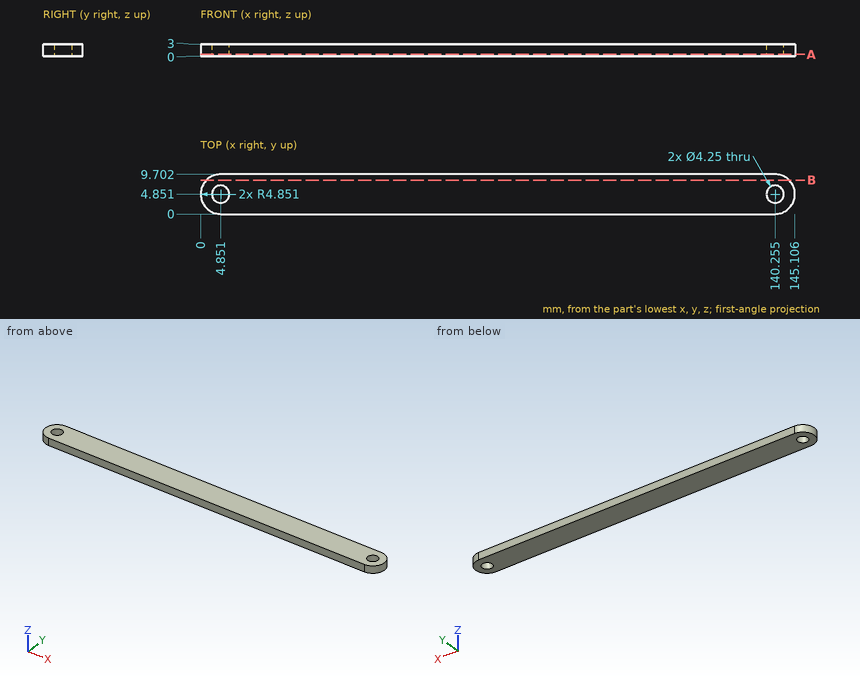
Print and shaded views of the part. All mm, measured from the part's lowest x, y and z. Give positions to 0.01 mm unless a question says otherwise; leave off trailing zeros. Loops run counter-clockwise (first coordinate to the right, second up) from the corner with the lowest first, then second, coordinate; pieces in that order, holes last. Notation, with made-up numbers: (11, 34.5) -> (25, 34.5) arc R31 cw to (25, 71.5) -> close; hole circle Ø5 at (-29.75, -5). An arc over 180 degrees is marked (long way). One line per question, with ' | ' between items. Start each with the question number.
1) Cut at A-A (z = 0.45). Count the separate pieces of the cut face and the enclosed holes in it, plus the area to 3 significant figures.
2) Cut at B-B (y = 8.25). Give the cut face in (x, z).
3) Pin check, flat tip, straight feed: pin 1 (3.5 mm diameter, centred on x = 140.26, y = 4.85, fed in from -Z). Stop position of the tip, or through.
4) Probe L1, parallel to X at y = 5, z = 0.5 (1 decimal); L2, parallel to X at y = 5.25, z = 0.2; L3, parallel to X at y = 0.5, z = 2.6 (1 decimal). List the from-to ranges inside material, lowest first.
Return value:
1) separate pieces: 1 | enclosed holes: 2 | area: 1,360 mm^2
2) outline: (1.39, 0) -> (143.72, 0) -> (143.72, 3) -> (1.39, 3) -> close
3) pin 1: through
4) L1: 0 to 2.7, 7 to 138.1, 142.4 to 145.1 | L2: 0.02 to 2.76, 6.94 to 138.17, 142.34 to 145.09 | L3: 2.7 to 142.4
